Verification items for the finished model (mm, model axes). Face numbers are marked on the shaded views. Coordinates: 2 decimals unless noted, no trailing zeros. Write each loop counter-clockwise with the first axis right and the second up, starting at its lowest first coordinate (ties: lowest second). Pieces come first, ordered by that corner, then holes.
```python
from build123d import *

# Parameters (mm, degrees)
SKETCH1_W           = 116
SKETCH1_H           = 48
BOSS_EXTRUDE1_DEPTH = 4
SKETCH2_R           = 2.5
CUT_EXTRUDE1_DEPTH  = 4
SKETCH3_W           = 44
SKETCH3_H           = 42
CUT_EXTRUDE2_DEPTH  = 4
SKETCH4_W           = 36
SKETCH4_H           = 4
BOSS_EXTRUDE2_DEPTH = 20
SKETCH5_W           = 116
SKETCH5_H           = 4
BOSS_EXTRUDE3_DEPTH = 6
CHAMFER1_SIZE       = 20
SKETCH6_R           = 5
BOSS_EXTRUDE4_DEPTH = 6
SKETCH7_R           = 2.25
CUT_EXTRUDE3_DEPTH  = 10


with BuildPart() as part:
    # Sketch1 → Boss-Extrude1 (new body)
    with BuildSketch(Plane(origin=(0, 0, 0), x_dir=(1, 0, 0), z_dir=(0, 1, 0))):
        Rectangle(SKETCH1_W, SKETCH1_H)
    extrude(amount=BOSS_EXTRUDE1_DEPTH)

    # Sketch2 → Cut-Extrude1 (cut)
    with BuildSketch(Plane(origin=(0, 4, 0), x_dir=(1, 0, 0), z_dir=(0, 1, 0))):
        with Locations(Location((-38, -2, 0), (0, 0, 270))):
            Circle(SKETCH2_R)
        with Locations(Location((38, -2, 0), (0, 0, 270))):
            Circle(SKETCH2_R)
    extrude(amount=-CUT_EXTRUDE1_DEPTH, mode=Mode.SUBTRACT)

    # Sketch3 → Cut-Extrude2 (cut)
    with BuildSketch(Plane(origin=(0, 4, 0), x_dir=(1, 0, 0), z_dir=(0, 1, 0))):
        with Locations((0, -3)):
            Rectangle(SKETCH3_W, SKETCH3_H)
    extrude(amount=-CUT_EXTRUDE2_DEPTH, mode=Mode.SUBTRACT)

    # Sketch4 → Boss-Extrude2 (add)
    with BuildSketch(Plane.XY.offset(24)):
        with Locations((-40, 2)):
            Rectangle(SKETCH4_W, SKETCH4_H)
        with Locations((40, 2)):
            Rectangle(SKETCH4_W, SKETCH4_H)
    extrude(amount=BOSS_EXTRUDE2_DEPTH)

    # Sketch5 → Boss-Extrude3 (add)
    with BuildSketch(Plane(origin=(0, 0, -24), x_dir=(-1, 0, 0), z_dir=(0, 0, -1))):
        with Locations((0, 2)):
            Rectangle(SKETCH5_W, SKETCH5_H)
    extrude(amount=BOSS_EXTRUDE3_DEPTH)

    # Chamfer1
    chamfer1_edges = [part.edges().sort_by_distance(p)[0] for p in [
        (-58, 2, 44),
        (58, 2, 44),
        (58, 2, -30),
        (-58, 2, -30),
    ]]
    chamfer(chamfer1_edges, length=CHAMFER1_SIZE)

    # Sketch6 → Boss-Extrude4 (add)
    with BuildSketch(Plane(origin=(0, 4, 0), x_dir=(1, 0, 0), z_dir=(0, 1, 0))):
        with Locations(Location((-35.928932188, 25, 0), (0, 0, 90))):
            Circle(SKETCH6_R)
        with Locations(Location((35.928932188, 25, 0), (0, 0, 90))):
            Circle(SKETCH6_R)
        with Locations(Location((35.928932188, -39, 0), (0, 0, 270))):
            Circle(SKETCH6_R)
        with Locations(Location((-35.928932188, -39, 0), (0, 0, 270))):
            Circle(SKETCH6_R)
    extrude(amount=BOSS_EXTRUDE4_DEPTH)

    # Sketch7 → Cut-Extrude3 (cut)
    with BuildSketch(Plane(origin=(0, 10, 0), x_dir=(1, 0, 0), z_dir=(0, 1, 0))):
        with Locations(Location((-35.928932188, 25, 0), (0, 0, 270))):
            Circle(SKETCH7_R)
        with Locations(Location((35.928932188, 25, 0), (0, 0, 270))):
            Circle(SKETCH7_R)
        with Locations(Location((35.928932188, -39, 0), (0, 0, 270))):
            Circle(SKETCH7_R)
        with Locations(Location((-35.928932188, -39, 0), (0, 0, 270))):
            Circle(SKETCH7_R)
    extrude(amount=-CUT_EXTRUDE3_DEPTH, mode=Mode.SUBTRACT)


solid = part.part
```
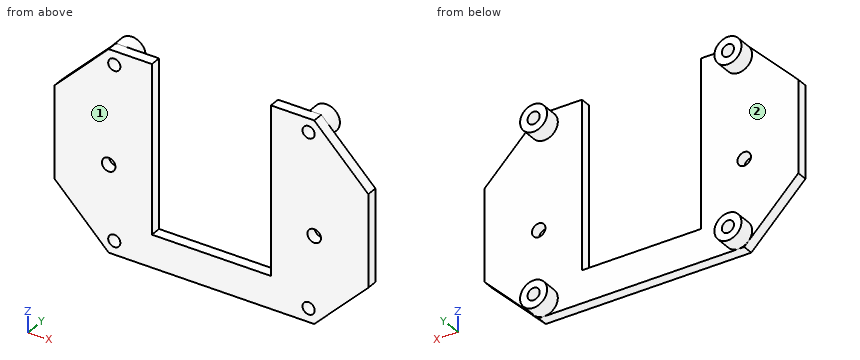
1. Sectioned sample at A-A, the plane z = 17.5. Record the boundary of the cut face in (x, y), and give its area (3 significant figures).
2. Sectioned sample at D-D, the plane z = -25. Record the boundary of the cut face in (x, y), and give its area (3 significant figures).
3. Material ranges on L1, parallel to X at y = 6.5, z = 39; L2, parallel to X at y = 1.4, z = 2; L3, parallel to X at y = 2, z = -25, recorded low to high.
4. Draft check along Z on the marked faces 1 and 2. Enter one of: pulls with the +Z half, pulls with the -Z half, needs draft (parallel to the pull), parting line crosses it, or undercut.
5. Sectioned sample at B-B, the plane y = 8.25. Record the boundary of the cut face in (x, z), and give its area (3 significant figures).
6. Sectioned sample at C-C, the plane z = 39. Record the boundary of the cut face in (x, y), and give its area (3 significant figures).
7. Gauge pin test, flat ends, axial feed: P1, Ø22, axis at x = -22.5, z = 21.5, coming from the +Y side; P2, Ø2, axis at x = -0.5, y = 1.5, coming from the +Z side; P3, Ø6, axis at x = -35.93, z = -25, coming from the +Y side; P4, Ø3, axis at x = 32, y = 6, coming from the -Z side. Record the tip position at first contact, or that the pin passes through.
Outcome:
1. outline: (-58, 0) - (-22, 0) - (-22, 4) - (-58, 4) - close; (22, 0) - (58, 0) - (58, 4) - (22, 4) - close
1. area: 288 mm2
2. outline: (-43, 0) - (-38.18, 0) - (-38.18, 10) - (-40.93, 10) - (-40.93, 4) - (-43, 4) - close; (-33.68, 0) - (33.68, 0) - (33.68, 10) - (30.93, 10) - (30.93, 4) - (-30.93, 4) - (-30.93, 10) - (-33.68, 10) - close; (38.18, 0) - (43, 0) - (43, 4) - (40.93, 4) - (40.93, 10) - (38.18, 10) - close
2. area: 374 mm2
3. L1: x = -40.93 to -38.18, -33.68 to -30.93, 30.93 to 33.68, 38.18 to 40.93
3. L2: x = -58 to -40.5, -35.5 to -22, 22 to 35.5, 40.5 to 58
3. L3: x = -43 to -38.18, -33.68 to 33.68, 38.18 to 43
4. face 1: needs draft
4. face 2: undercut
5. outline: circle Ø10 at (-35.93, -25); circle Ø10 at (-35.93, 39); circle Ø10 at (35.93, -25); circle Ø10 at (35.93, 39); hole circle Ø4.5 at (-35.93, -25); hole circle Ø4.5 at (-35.93, 39); hole circle Ø4.5 at (35.93, -25); hole circle Ø4.5 at (35.93, 39)
5. area: 251 mm2
6. outline: (-43, 0) - (-38.18, 0) - (-38.18, 10) - (-40.93, 10) - (-40.93, 4) - (-43, 4) - close; (-33.68, 0) - (-22, 0) - (-22, 4) - (-30.93, 4) - (-30.93, 10) - (-33.68, 10) - close; (22, 0) - (33.68, 0) - (33.68, 10) - (30.93, 10) - (30.93, 4) - (22, 4) - close; (38.18, 0) - (43, 0) - (43, 4) - (40.93, 4) - (40.93, 10) - (38.18, 10) - close
6. area: 198 mm2
7. P1: stops at y = 4
7. P2: stops at z = -18
7. P3: stops at y = 10
7. P4: stops at z = -29.37
